from build123d import *

# Parameters (mm, degrees)
SKETCH1_W           = 140
SKETCH1_H           = 40
BOSS_EXTRUDE1_DEPTH = 3
SKETCH2_R           = 1.4
SKETCH2_R_2         = 1.25
SKETCH2_R_3         = 1.45
CUT_EXTRUDE1_DEPTH  = 146.633100633
CUT_EXTRUDE2_DEPTH  = 2.5
SKETCH5_W           = 46.87
SKETCH5_H           = 9.866874784
CUT_EXTRUDE4_DEPTH  = 146.633100633


with BuildPart() as part:
    # Sketch1 → Boss-Extrude1 (new body)
    with BuildSketch(Plane(origin=(0, 0, 0), x_dir=(1, 0, 0), z_dir=(0, 1, 0))):
        with Locations((70, 20)):
            Rectangle(SKETCH1_W, SKETCH1_H)
    extrude(amount=BOSS_EXTRUDE1_DEPTH)

    # Sketch2 → Cut-Extrude1 (cut, through all)
    with BuildSketch(Plane.XZ):
        with Locations(Location((3.675, -35, 0), (0, 0, 270))):
            Circle(SKETCH2_R)
        with Locations(Location((21.325, -35, 0), (0, 0, 270))):
            Circle(SKETCH2_R)
        with Locations(Location((5.95, -3.8, 0), (0, 0, 270))):
            Circle(SKETCH2_R_2)
        with Locations(Location((19.05, -3.8, 0), (0, 0, 270))):
            Circle(SKETCH2_R_2)
        with Locations(Location((36.32, -33.85, 0), (0, 0, 270))):
            Circle(SKETCH2_R_3)
        with Locations(Location((52.42, -33.85, 0), (0, 0, 270))):
            Circle(SKETCH2_R_3)
        with Locations(Location((52.42, -16.15, 0), (0, 0, 270))):
            Circle(SKETCH2_R_3)
        with Locations(Location((36.32, -16.15, 0), (0, 0, 270))):
            Circle(SKETCH2_R_3)
        with Locations(Location((75.545, -35, 0), (0, 0, 270))):
            Circle(SKETCH2_R)
        with Locations(Location((93.195, -35, 0), (0, 0, 270))):
            Circle(SKETCH2_R)
        with Locations(Location((77.82, -3.8, 0), (0, 0, 270))):
            Circle(SKETCH2_R_2)
        with Locations(Location((90.92, -3.8, 0), (0, 0, 270))):
            Circle(SKETCH2_R_2)
        with Locations(Location((102.342999781, -33.85, 0), (0, 0, 270))):
            Circle(SKETCH2_R_3)
        with Locations(Location((118.442999781, -33.85, 0), (0, 0, 270))):
            Circle(SKETCH2_R_3)
        with Locations(Location((102.342999781, -16.15, 0), (0, 0, 270))):
            Circle(SKETCH2_R_3)
        with Locations(Location((118.442999781, -16.15, 0), (0, 0, 270))):
            Circle(SKETCH2_R_3)
    extrude(amount=-CUT_EXTRUDE1_DEPTH, mode=Mode.SUBTRACT)

    # Sketch3 → Cut-Extrude2 (cut)
    with BuildSketch(Plane.XZ):
        Polygon((8, -4.983568052), (8, -2.616431948), (5.95, -1.432863896), (3.9, -2.616431948), (3.9, -4.983568052), (5.95, -6.167136104), align=None)
        Polygon((21.1, -4.983568052), (21.1, -2.616431948), (19.05, -1.432863896), (17, -2.616431948), (17, -4.983568052), (19.05, -6.167136104), align=None)
        Polygon((6.325, -36.529978213), (6.325, -33.470021787), (3.675, -31.940043573), (1.025, -33.470021787), (1.025, -36.529978213), (3.675, -38.059956427), align=None)
        Polygon((21.325, -38.059956427), (23.975, -36.529978213), (23.975, -33.470021787), (21.325, -31.940043573), (18.675, -33.470021787), (18.675, -36.529978213), align=None)
        Polygon((38.97, -17.679978213), (38.97, -14.620021787), (36.32, -13.090043573), (33.67, -14.620021787), (33.67, -17.679978213), (36.32, -19.209956427), align=None)
        Polygon((52.42, -19.209956427), (55.07, -17.679978213), (55.07, -14.620021787), (52.42, -13.090043573), (49.77, -14.620021787), (49.77, -17.679978213), align=None)
        Polygon((38.97, -35.379978213), (38.97, -32.320021787), (36.32, -30.790043573), (33.67, -32.320021787), (33.67, -35.379978213), (36.32, -36.909956427), align=None)
        Polygon((55.07, -35.379978213), (55.07, -32.320021787), (52.42, -30.790043573), (49.77, -32.320021787), (49.77, -35.379978213), (52.42, -36.909956427), align=None)
        Polygon((78.195, -33.470021787), (75.545, -31.940043573), (72.895, -33.470021787), (72.895, -36.529978213), (75.545, -38.059956427), (78.195, -36.529978213), align=None)
        Polygon((95.845, -36.529978213), (95.845, -33.470021787), (93.195, -31.940043573), (90.545, -33.470021787), (90.545, -36.529978213), (93.195, -38.059956427), align=None)
        Polygon((90.92, -6.167136104), (92.97, -4.983568052), (92.97, -2.616431948), (90.92, -1.432863896), (88.87, -2.616431948), (88.87, -4.983568052), align=None)
        Polygon((79.87, -4.983568052), (79.87, -2.616431948), (77.82, -1.432863896), (75.77, -2.616431948), (75.77, -4.983568052), (77.82, -6.167136104), align=None)
        Polygon((118.442999781, -30.790043573), (115.792999781, -32.320021787), (115.792999781, -35.379978213), (118.442999781, -36.909956427), (121.092999781, -35.379978213), (121.092999781, -32.320021787), align=None)
        Polygon((102.342999781, -30.790043573), (99.692999781, -32.320021787), (99.692999781, -35.379978213), (102.342999781, -36.909956427), (104.992999781, -35.379978213), (104.992999781, -32.320021787), align=None)
        Polygon((102.342999781, -13.090043573), (99.692999781, -14.620021787), (99.692999781, -17.679978213), (102.342999781, -19.209956427), (104.992999781, -17.679978213), (104.992999781, -14.620021787), align=None)
        Polygon((118.442999781, -13.090043573), (115.792999781, -14.620021787), (115.792999781, -17.679978213), (118.442999781, -19.209956427), (121.092999781, -17.679978213), (121.092999781, -14.620021787), align=None)
    extrude(amount=-CUT_EXTRUDE2_DEPTH, mode=Mode.SUBTRACT)

    # Sketch5 → Cut-Extrude4 (cut, through all)
    with BuildSketch(Plane(origin=(0, 3, 0), x_dir=(1, 0, 0), z_dir=(0, 1, 0))):
        with Locations((48.435, 4.933437392)):
            Rectangle(SKETCH5_W, SKETCH5_H)
        Polygon((96.87, 9.866874784), (122.892999781, 9.866874784), (122.892999781, 40), (140, 40), (140, 9.866874784), (140, 0), (96.87, 0), align=None)
    extrude(amount=-CUT_EXTRUDE4_DEPTH, mode=Mode.SUBTRACT)


solid = part.part
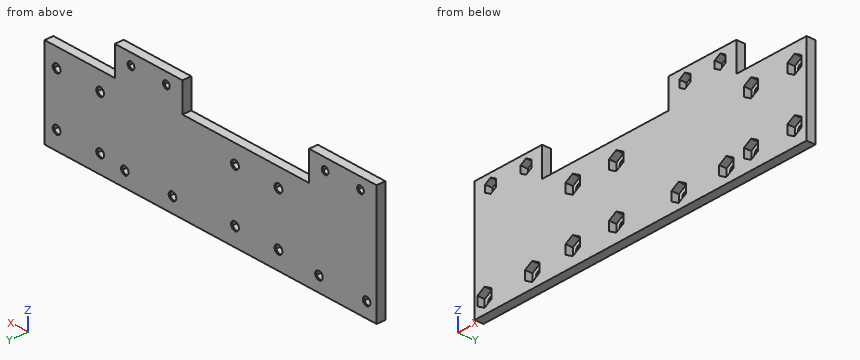
Model file for the job. Use its own axes, mm. Coordinates: 2 decimals unless noted, no trailing zeros. Write each loop counter-clockwise with the first axis right and the second up, starting at its lowest first coordinate (ties: lowest second). Pieces come first, ordered by that corner, then holes. Notation, with made-up numbers: (-10, -19.5) - (-6, -19.5) arc R7 cw to (-6, -10.5) - close; hole circle Ø7 at (-2.5, -3). An arc over 180 degrees is marked (long way). Write each question's results on one line, items separated by ' | '. Start each with the question number.
1) Probe line 1 along X through (y, z) = (2.7, -3.8); line 2 along X through (y, z) = (2.4, -31.5); line 3 along X through (y, z) = (0.7, -5). List the from-to ranges inside material, lowest first. Write a range as from..to.
2) Cut at C-C (x = 112.5). Write the cut outline in (y, z), then the cut area to 3 significant figures.
3) Cut at B-B (y = 1.7). Count the separate pieces of the cut face and the enclosed holes in it, then the cut area to 3 significant figures.
4) Flat gauge pins, fed straight in: P1, Ø1.2, axis at y = 1.5, z = -34, coming from the -X side; P2, Ø1.6, axis at x = 119.5, z = -15, coming from the -Y side; P3, Ø0.7, axis at y = 1.5, z = -4, coming from the +X side. Where does each tip first touch, or does it go through?
5) Cut at A-A (z = -8). Write the cut outline in (x, y).
Returned:
1) line 1: 0..4.7, 7.2..17.8, 20.3..25, 71.87..76.57, 79.07..89.67, 92.17..96.87 | line 2: 0..35.09, 37.55..51.19, 53.65..101.11, 103.57..117.21, 119.67..122.89 | line 3: 0..3.93, 7.97..17.03, 21.07..25, 71.87..75.8, 79.84..88.9, 92.94..96.87
2) outline: (0, -40) - (3, -40) - (3, -9.87) - (0, -9.87) - close | area: 90.4 mm^2
3) separate pieces: 1 | enclosed holes: 16 | area: 3,850 mm^2
4) P1: x = 0 | P2: y = 2.5 | P3: x = 96.87
5) outline: (0, 0) - (25, 0) - (25, 3) - (0, 3) - close; (71.87, 0) - (96.87, 0) - (96.87, 3) - (71.87, 3) - close
